Verification items for the finished model (mm, model axes). A direction names the side the tool comes from. Coordinates: 2 decimals unless noted, no trailing zeros. Write each loop counter-clockwise with the first axis right and the second up, starting at its lowest first coordinate (ties: lowest second). Pieces come first, ordered by that corner, then holes. Notation, with made-up numbers: M 55.5,72 L 82.5,72 A9 cw 82.5,76 Z; hole C -26,11.25 d6. An arc over 180 degrees is marked long. Answer in a Markdown table with one row per item.
from build123d import *

# Parameters (mm, degrees)
F0_W      = 130
F0_H      = 50
F1_DEPTH  = 150
F2_W      = 75
F2_H      = 25.0761986731
F3_DEPTH  = 130.001
F6_DEPTH  = 25
F8_DEPTH  = 25
F10_DEPTH = 25
F11_W     = 150
F11_H     = 15
F12_DEPTH = 161
F13_W     = 20
F13_H     = 75
F13_W_2   = 29.982657928
F13_W_3   = 30.0133985095
F13_W_4   = 19.9825553596
F14_DEPTH = 25
F15_W     = 75
F15_H     = 9.9238013269
F16_DEPTH = 100
F17_R     = 2
F18_DEPTH = 10
F19_W     = 55
F19_H     = 25
F20_DEPTH = 140
F4_W      = 10
F4_H      = 75
F21_DEPTH = 25


with BuildPart() as f1:
    # F0 (on Front) → F1 (new body)
    with BuildSketch(Plane.XZ):
        with Locations((0.7955543697, 0.0761986731)):
            Rectangle(F0_W, F0_H)
    extrude(amount=F1_DEPTH)

    # F2 (on face) → F3 (cut, through all)
    with BuildSketch(Plane.YZ.offset(65.7955543697)):
        with Locations((-37.5, 12.5380993366)):
            Rectangle(F2_W, F2_H)
    extrude(amount=-F3_DEPTH, mode=Mode.SUBTRACT)

    # F5 (on face) → F6 (cut)
    with BuildSketch(Plane.XY.offset(25.0761986731)):
        Polygon((-31.2077699304, -75), (-47.2077699304, -75), (-47.2077699304, -80.0817286968), (-53.221039474, -80.0817286968), (-53.221039474, -82.5817286968), (-47.2077699304, -82.5817286968), (-47.2077699304, -145.5817286968), (-42.0114186667, -148.5818434977), (-42.0114186667, -150), (-36.4380876982, -150), (-36.4078128177, -148.5839748576), (-31.2077699304, -145.5817286968), (-31.2077699304, -82.5817286968), (-25.2643544227, -82.5817286968), (-25.2643544227, -80.0817286968), (-31.2077699304, -80.0817286968), align=None)
    extrude(amount=-F6_DEPTH, mode=Mode.SUBTRACT)

    # F7 (on face) → F8 (cut)
    with BuildSketch(Plane.XY.offset(25.0761986731)):
        Polygon((48.7916108072, -73.9334896207), (32.7916108072, -73.8659650087), (32.7916108072, -79.9098435044), (26.7916108072, -79.9098435044), (26.7916108072, -82.4098435044), (32.7916108072, -82.4098435044), (32.7916108072, -145.4098435044), (37.9877632299, -148.4098435044), (37.9877632299, -152.647121688), (43.5954583845, -152.647121688), (43.5954583845, -148.4773681164), (48.7916108072, -145.4773681164), (48.7916108072, -82.4773681164), (54.7916108072, -82.4773681164), (54.7916108072, -79.9773681164), (48.7916108072, -79.9773681164), align=None)
    extrude(amount=-F8_DEPTH, mode=Mode.SUBTRACT)

    # F9 (on face) → F10 (cut)
    with BuildSketch(Plane.XY.offset(25.0761986731)):
        Polygon((8.7782122977, -73.7298429012), (-7.2217877023, -73.7298429012), (-7.2217877023, -79.9959796667), (-13.2217877023, -79.9959796667), (-13.2217877023, -82.4959796667), (-7.2217877023, -82.4959796667), (-7.2217877023, -145.4959796667), (-2.0256352796, -148.4959796667), (-2.0256352796, -153.1414538622), (3.6333000753, -153.1414538622), (3.582059875, -148.4959796667), (8.7782122977, -145.4959796667), (8.7782122977, -82.4959796667), (14.7782122977, -82.4959796667), (14.7782122977, -79.9959796667), (8.7782122977, -79.9959796667), align=None)
    extrude(amount=-F10_DEPTH, mode=Mode.SUBTRACT)

    # F11 (on face) → F12 (cut)
    with BuildSketch(Plane.YZ.offset(65.7955543697)):
        with Locations((-75, -17.4238013269)):
            Rectangle(F11_W, F11_H)
    extrude(amount=-F12_DEPTH, mode=Mode.SUBTRACT)

    # F13 (on face) → F14 (cut)
    with BuildSketch(Plane.XY):
        with Locations((-54.2044456303, -37.5)):
            Rectangle(F13_W, F13_H)
        with Locations((-19.2131166663, -37.5)):
            Rectangle(F13_W_2, F13_H)
        with Locations((20.7849115524, -37.5)):
            Rectangle(F13_W_3, F13_H)
        with Locations((55.8042766899, -37.5)):
            Rectangle(F13_W_4, F13_H)
    extrude(amount=-F14_DEPTH, mode=Mode.SUBTRACT)

    # F15 (on face) → F16 (cut)
    with BuildSketch(Plane.YZ.offset(45.8129990101)):
        with Locations((-37.5, -4.9619006634)):
            Rectangle(F15_W, F15_H)
    extrude(amount=-F16_DEPTH, mode=Mode.SUBTRACT)

    # F17 (on face) → F18 (cut)
    with BuildSketch(Plane(origin=(0, -75, 0), x_dir=(-1, 0, 0), z_dir=(0, 1, 0))):
        with Locations((-40.7916108072, -4.9238013269)):
            Circle(F17_R)
        with Locations((-0.7782122977, -4.9238013269)):
            Circle(F17_R)
        with Locations((39.2077699304, -4.9238013269)):
            Circle(F17_R)
    extrude(amount=-F18_DEPTH, mode=Mode.SUBTRACT)

    # F19 (on face) → F20 (cut)
    with BuildSketch(Plane.YZ.offset(65.7955543697)):
        with Locations((-113.85, 12.5761986731)):
            Rectangle(F19_W, F19_H)
    extrude(amount=-F20_DEPTH, mode=Mode.SUBTRACT)

    # F4 (on face) → F21 (cut)
    with BuildSketch(Plane.XY.offset(25.0761986731)):
        with Locations((-19.2044456303, -112.5)):
            Rectangle(F4_W, F4_H)
        with Locations((20.7955543697, -112.5)):
            Rectangle(F4_W, F4_H)
    extrude(amount=-F21_DEPTH, mode=Mode.SUBTRACT)


solid = f1.part
1) Tool access check on faces 1 (the face through (25.796, -81, 13)), 2 (the face through (-56, -86.35, 12)), 3 (the face through (52, -79.977, 13)), 4 (the face through (-7.222, -77, 13)). Record the directions out of +Z, -Z, +X, -X, +Y, -Y that give a thin tool (end or side, any length) a straight path to the whole face; none if there is none.
Response values:
| item | result |
|---|---|
| face 1 | +Z, +Y, -Y |
| face 2 | +Z, +X, -X |
| face 3 | +Z |
| face 4 | +Z, +Y |
2) Depth check by flat-ended pin: pin 1 (6 mm diameter, centred on x = 23.5, y = -121.5, fed in from +Z); pin 2 (5 mm diameter, centred on x = 22.5, z = 7, fed in from -Y). Enter the tip coordinate at first touch or a pass-through.
Response values:
| item | result |
|---|---|
| pin 1 | stops at z = 0.08 |
| pin 2 | passes through |
3) Release check for a two-part mould opening along X. For faces 5 (the face through (-11, -141.35, 12)), 6 (the face through (-64.204, -112, -0.4)), 7 (the face through (41, -85, -5)) record: +X half, -X half, draft (parallel to the pull), parting line (faces both ways), or undercut.
Response values:
| item | result |
|---|---|
| face 5 | draft |
| face 6 | -X half |
| face 7 | undercut |
4) Sectioned sample at C-C (x = 47.5). Record the cut outline in (y, z).
Response values:
| item | result |
|---|---|
| outline | M -150,-9.92 L -75,-9.92 L -75,0.08 L -146.22,0.08 L -146.22,25.08 L -150,25.08 Z |
5) Sectioned sample at A-A (z = 5). Give the number of separate pieces and of enclosed holes in the cut face, then the cut area to 3 significant figures.
Response values:
| item | result |
|---|---|
| separate pieces | 12 |
| enclosed holes | 0 |
| area | 1,240 mm² |
6) Sectioned sample at B-B (y = -119). Record the cut outline in (x, z), then the cut area to 3 significant figures.
Response values:
| item | result |
|---|---|
| outline | M -64.2,-9.92 L 65.8,-9.92 L 65.8,0.08 L -64.2,0.08 Z |
| area | 1,300 mm² |
7) Thickness scan on L1, parallel to X at y = -83, z = 23; L2, parallel to Y at x = 13, z = 3; L3, parallel to Y at x = 29, z = 9.5. Record the ranges inside material, lowest first. Write a range as [from, to].
Response values:
| item | result |
|---|---|
| L1 | x = [-64.2, -47.21], [-31.21, -24.2], [-14.2, -7.22], [8.78, 15.8], [25.8, 32.79], [48.79, 65.8] |
| L2 | y = [-150, -141.35], [-86.35, -82.5], [-80, -75] |
| L3 | y = [-150, -141.35], [-86.35, -82.41], [-79.91, -75] |
8) Sectioned sample at D-D (x = 21). Record the cut outline in (y, z).
Response values:
| item | result |
|---|---|
| outline | M -150,-9.92 L -75,-9.92 L -75,0.08 L -150,0.08 Z |
